Autodesk Inventor part; units mm, degrees
ref_plane "YZ Plane" through (0, 0, 0) normal (1, 0, 0) x (0, 1, 0)
ref_plane "XZ Plane" through (0, 0, 0) normal (0, 1, 0) x (-1, 0, 0)
ref_plane "XY Plane" through (0, 0, 0) normal (0, 0, 1) x (1, 0, 0)
sketch "Sketch1" plane through (0, 0, 0) normal (0, 0, 1) x (1, 0, 0)
  line L0 (-50, -50) -> (50, -50)
  line L1 (50, -50) -> (50, 50)
  line L2 (50, 50) -> (-50, 50)
  line L3 (-50, 50) -> (-50, -50)
  line L4 (-50, -50) -> (50, 50) construction
  line L5 (50, -50) -> (-50, 50) construction
  point P0 (0, 0)
  dimension "d0" = 100
  dimension "d1" = 100
extrude "Extrusion1" add sketch "Sketch1" along normal blind 3
sketch "Sketch2" plane through (-50, 50, 0) normal (0, 1, 0) x (1, 0, 0)
  line L0 (0, 0) -> (100, 0)
  line L1 (0, 0) -> (50, 50)
  line L2 (50, 50) -> (52.1213, 47.8787)
  line L3 (52.1213, 47.8787) -> (2.1213, -2.1213)
  line L4 (2.1213, -2.1213) -> (0, 0)
  line L5 (0, 0) -> (70.7107, 0) construction
  line L6 (100, 0) -> (52.1213, 47.8787)
  line L7 (52.1213, 47.8787) -> (50, 45.7574)
  line L8 (50, 45.7574) -> (97.8787, -2.1213)
  line L9 (97.8787, -2.1213) -> (100, 0)
  point P0 (50, 0)
  dimension "d4" = 45
  dimension "d5" = 3
  dimension "d6" = 3
extrude "Extrusion2" add sketch "Sketch2" against normal blind 55 contours L1 L2 L3 L0 | L0 L3 L4 | L8 L3 L6 L0 | L0 L9 L8
sketch "Sketch3" plane through (0, 0, 3) normal (0, 0, 1) x (1, 0, 0)
  line L0 (2.5, -25) -> (-2.5, -25)
  line L1 (-17.5, -10) -> (-17.5, 10)
  line L2 (-2.5, 25) -> (2.5, 25)
  line L3 (17.5, 10) -> (17.5, -10)
  line L4 (17.5, -25) -> (-17.5, 25) construction
  line L5 (-17.5, -25) -> (17.5, 25) construction
  arc A0 (-2.5, 25) -> (-17.5, 10) centre (-2.5, 10) ccw
  arc A1 (17.5, 10) -> (2.5, 25) centre (2.5, 10) ccw
  arc A2 (2.5, -25) -> (17.5, -10) centre (2.5, -10) ccw
  arc A3 (-17.5, -10) -> (-2.5, -25) centre (-2.5, -10) ccw
  point P0 (0, 0)
  dimension "d9" = 35
  dimension "d10" = 50
  dimension "d11" = 15
extrude "Extrusion3" cut sketch "Sketch3" against normal blind 3
sketch "Sketch4" plane through (-50, 50, 3) normal (0, 1, 0) x (1, 0, 0)
  line L0 (95.7574, 3) -> (50, 48.7574)
  line L1 (95.7574, 3) -> (4.2426, 3)
  line L2 (50, 48.7574) -> (4.2426, 3)
  line L3 (95.7574, 3) -> (100, 3)
  line L4 (4.2426, 3) -> (95.7574, 3)
  line L5 (95.7574, 3) -> (50, 48.7574)
  line L6 (0, 3) -> (50, 53)
  point P0 (50, 3)
extrude "Extrusion4" add sketch "Sketch4" against normal blind 3
properties part number "fixation"
Work out the finished part from the listing and answer in its coordinate system (mm). A direction names the side the tool comes from. Coordinates: 2 decimals unless noted, no trailing zeros. Order: outer loops, then holes, each group sorted by start corner. A loop starts at its lowest first (then second) coordinate and runs counter-clockwise, first axis right, second up. Notation, with made-up numbers: (65.25, 58.25) - (123.25, 58.25) arc R30 ccw to (123.25, 95.25) - close; hole circle Ø1 at (-33, 22.25). An arc over 180 degrees is marked (long way). Answer as a JSON object with one key per item and string values.
1. Find section A-A on y = 34. Determine the outline of the cut face in (x, z).
Output values:
{"outline": "(-50, 0) - (0, -50) - (50, 0) - (50, 3) - (-50, 3) - close; hole (-45.76, 0) - (0, -45.76) - (45.76, 0) - close"}
2. Find section C-C on x = 14.5. Determine the outline of the cut face in (y, z).
Output values:
{"outline": "(-50, 0) - (-19, 0) - (-19, 3) - (-50, 3) - close; (-5, -35.5) - (50, -35.5) - (50, 3) - (19, 3) - (19, 0) - (47, 0) - (47, -31.26) - (-5, -31.26) - close"}
3. Consider line 1 (Z direction, x = -14.5, y = -43); line 2 (X direction, y = 44, z = -5); line 3 (Y direction, x = -18.5, z = -13). Determine where each line is inside the solid, lowest interval first.
Output values:
{"line 1": "z = 0 to 3", "line 2": "x = -45 to -40.76, 40.76 to 45", "line 3": "y = 47 to 50"}
4. The mould has two halves that part along X. Classify faces 1 (the face through (25, 23, -25)), 2 (the face through (-1, -50, 1)), 3 (the face through (-17.5, 0, 2)): +X half, -X half, draft (parallel to the pull), parting line (faces both ways), or undercut.
Output values:
{"face 1": "+X half", "face 2": "draft", "face 3": "undercut"}
5. Find section D-D on z = -37. Determine the outline of the cut face in (x, y).
Output values:
{"outline": "(-13, -5) - (-8.76, -5) - (-8.76, 47) - (8.76, 47) - (8.76, -5) - (13, -5) - (13, 50) - (-13, 50) - close"}
6. Find section B-B on y = -21. Determine the outline of the cut face in (x, z), plus the area to 3 significant figures.
Output values:
{"outline": "(-50, 0) - (-12.7, 0) - (-12.7, 3) - (-50, 3) - close; (12.7, 0) - (50, 0) - (50, 3) - (12.7, 3) - close", "area": "224 mm²"}
7. This flat-tipped pin is pushed along its axis until it touches: P1, Ø12, axis at x = -23.5, z = -26, coming from the -Y side. Where does it stop, or does it pass through?
Output values:
{"P1": "stops at y = -5"}
8. A tool of negligible diameter and unlimited length cuts with its end or side. For faces 4 (the face through (0, -25, 2)), 5 (the face through (13.22, 20.49, 1.52)), 6 (the face through (22.56, 21.36, -23.2)), from which of +Z, -Z, +X, -X, +Y, -Y can it reach the whole face along a straight path? Write none if from no direction.
Output values:
{"face 4": "+Z, -Z", "face 5": "+Z", "face 6": "-Y"}
